Geometry check sheet. Reference: the model listing, model coordinates, mm. Round coordinates to 2 decimals unless told otherwise and drop trailing zeros. Order: outer loops, then holes, each group sorted by start corner. A loop starts at its lowest first (then second) coordinate and runs counter-clockwise, first axis right, second up. Notation, with made-up numbers: (24.5, 23.5) - (57.5, 23.5) arc R12 ccw to (57.5, 32.5) - close; hole circle Ø6 at (19, -22.75). An arc over 180 degrees is marked (long way). Return JSON: item names as keys, results as strings. Group by question number.
Q1. Sectioned sample at C-C, the plane y = 49. Record the cut outline in (x, z), then the cut area to 3 significant figures.
Q2. Material ranges on line 1 along Z through (x, y) = (459, 98); line 2 along Y through (x, z) = (832.5, -34); line 3 along X through (y, z) = (93, -45), recorded low to high.
Q3. Sectioned sample at B-B, the plane z = -18. Record the cut outline in (x, y), then the cut area to 3 significant figures.
Q4. Gauge pin test, flat ends, axial feed: pin 1 Ø1 at (y, z) = (113.5, -28.5) entering from +X; pin 2 Ø10 at (y, z) = (15, -6) entering from -X; pin 3 Ø12 at (y, z) = (74.5, -32.5) entering from +X. Record the tip position at first contact, or that the pin passes through.
Q5. Sectioned sample at A-A, the plane x = 479. Record the cut outline in (y, z), then the cut area to 3 significant figures.
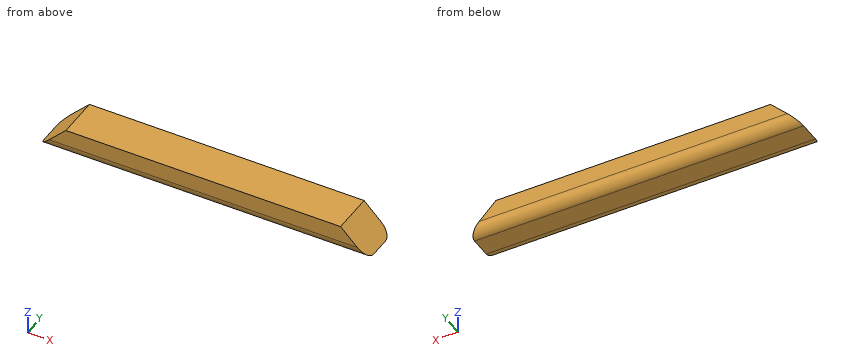
```python
from build123d import *

# Parameters (mm, degrees)
BOSS_EXTRUDE1_DEPTH = 996.95
SKETCH2_W           = 344.402501539
SKETCH2_H           = 493.213131915
CUT_EXTRUDE1_DEPTH  = 59.371664787


with BuildPart() as part:
    # Sketch1 → Boss-Extrude1 (new body)
    with BuildSketch(Plane(origin=(0, 0, 0), x_dir=(0, 0, -1), z_dir=(1, 0, 0))):
        with BuildLine():
            Line((0, 0), (31.75, 0))
            ThreePointArc((31.75, 0), (54.200640303, 9.299359697), (63.5, 31.75))
            Line((63.5, 31.75), (63.5, 95.25))
            ThreePointArc((63.5, 95.25), (54.200640303, 117.700640303), (31.75, 127))
            Line((31.75, 127), (0, 127))
            Line((0, 127), (-19.05, 127))
            Line((-19.05, 127), (-19.05, 0))
            Line((-19.05, 0), (0, 0))
        make_face()
    extrude(amount=BOSS_EXTRUDE1_DEPTH)

    # Sketch2 → Cut-Extrude1 (cut, through all)
    with BuildSketch(Plane(origin=(466.725, 0, 466.725), x_dir=(0, 1, 0), z_dir=(0.707106781, 0, 0.707106781))):
        with Locations((32.995160032, -679.680893327)):
            Rectangle(SKETCH2_W, SKETCH2_H)
    cut_extrude1 = extrude(amount=CUT_EXTRUDE1_DEPTH, mode=Mode.SUBTRACT)

    # Mirror1: Cut-Extrude1 across plane
    add(cut_extrude1.mirror(Plane(origin=(498.475, 0, 0), x_dir=(0, 0, 1), z_dir=(1, 0, 0))), mode=Mode.SUBTRACT)


solid = part.part
```
Reply:
{
 "1": {"outline": "(0, -63.5) - (996.95, -63.5) - (914.4, 19.05) - (82.55, 19.05) - close", "area": "75,500 mm^2"},
 "2": {"line 1": "-63.38 to 19.05", "line 2": "0.08 to 126.92", "line 3": "18.5 to 978.45"},
 "3": {"outline": "(45.5, 0) - (951.45, 0) - (951.45, 127) - (45.5, 127) - close", "area": "115,000 mm^2"},
 "4": {"pin 1": "x = 962.45", "pin 2": "x = 52.5", "pin 3": "x = 971.95"},
 "5": {"outline": "(0, -31.75) arc R31.75 ccw to (31.75, -63.5) - (95.25, -63.5) arc R31.75 ccw to (127, -31.75) - (127, 19.05) - (0, 19.05) - close", "area": "10,100 mm^2"}
}
